from build123d import *

# Parameters (mm, degrees)
F0_R         = 19.3201303499
F1_DEPTH     = 45.72
F2_T1_DEPTH  = 55.325963316
F2_T3_DEPTH  = 52.1146440054
F2_T5_DEPTH  = 66.4513256331
F2_T7_DEPTH  = 30.5870827045
F2_T9_DEPTH  = 100.2395855595
F2_T11_DEPTH = 63.3652483976
F2_T13_DEPTH = 70.2836609721
F2_T15_DEPTH = 91.0933305156
F2_T20_DEPTH = 5.08
F2_T26_DEPTH = 5.08
F2_T36_DEPTH = 59.2845010847
F2_T41_DEPTH = 57.568004282
F2_T46_DEPTH = 31.0915483116
F2_T51_DEPTH = 75.0016446771
F2_T57_DEPTH = 59.2845010847
F2_T61_DEPTH = 57.568004282
F2_T68_DEPTH = 31.0915483116
F2_T72_DEPTH = 75.0016446771


# Not quite as in the source:
# - a fillet or chamfer that OpenCascade refuses, or shapes differently, is made with other operations: its cross-section is extruded or revolved along the edge and cut away or added


with BuildPart() as f1:
    # F0 (on Top) → F1 (new body)
    with BuildSketch(Plane.XY):
        Polygon((13.1280273199, 53.9313554764), (-58.0116845667, 30.691197142), (-58.1890903413, -7.2736367583), (-24.3045892566, -7.2736367583), (-13.1280263886, -56.7698441446), (25.1916181296, -42.0451648533), (19.1598236561, -19.8694467545), (68.3012157679, -26.610866189), (68.3012157679, 18.2727947831), align=None)
        with Locations((-4.6125496738, 20.4016622156)):
            Circle(F0_R, mode=Mode.SUBTRACT)
    extrude(amount=F1_DEPTH)

    # F2: fillet of radius 5.08 on 15 edges, made by hand

    # F2_s2 → F2_t1 (cut)
    with BuildSketch(Plane.XY.offset(-14.685963316)):
        with BuildLine():
            ThreePointArc((-14.4219236098, -51.039727833), (-11.8616097658, -54.4008391443), (-7.6445406789, -54.662763834))
            Line((-7.6445406789, -54.662763834), (-13.1280263886, -56.7698441446))
            Line((-13.1280263886, -56.7698441446), (-14.4219236098, -51.039727833))
        make_face()
    extrude(amount=F2_T1_DEPTH, mode=Mode.SUBTRACT)

    # F2_s4 → F2_t3 (cut)
    with BuildSketch(Plane.XY.offset(-11.4746440054)):
        with BuildLine():
            ThreePointArc((20.9071837297, -43.6914985622), (23.6160955732, -41.2464799373), (23.9869451943, -37.6162196147))
            Line((23.9869451943, -37.6162196147), (25.1916181296, -42.0451648533))
            Line((25.1916181296, -42.0451648533), (20.9071837297, -43.6914985622))
        make_face()
    extrude(amount=F2_T3_DEPTH, mode=Mode.SUBTRACT)

    # F2_s6 → F2_t5 (cut)
    with BuildSketch(Plane(origin=(-42.3016489373, -16.2548014713, 0), x_dir=(0, 0, 1), z_dir=(0.9334569329, 0.3586894958, 0))):
        with BuildLine():
            ThreePointArc((5.08, 48.2833194327), (1.4878975516, 46.7954218811), (0, 43.2033194327))
            Line((0, 43.2033194327), (0, 48.2833194327))
            Line((0, 48.2833194327), (5.08, 48.2833194327))
        make_face()
    extrude(amount=F2_T5_DEPTH, mode=Mode.SUBTRACT)

    # F2_s8 → F2_t7 (cut)
    with BuildSketch(Plane(origin=(-24.9632601794, -9.5923645646, 0), x_dir=(0, 0, 1), z_dir=(0.9334569329, 0.3586894958, 0))):
        with BuildLine():
            ThreePointArc((40.64, 48.2833194327), (44.2321024484, 46.7954218811), (45.72, 43.2033194327))
            Line((45.72, 43.2033194327), (45.72, 48.2833194327))
            Line((45.72, 48.2833194327), (40.64, 48.2833194327))
        make_face()
    extrude(amount=F2_T7_DEPTH, mode=Mode.SUBTRACT)

    # F2_s10 → F2_t9 (cut)
    with BuildSketch(Plane(origin=(39.8537401384, 13.0195527431, 0), x_dir=(0, 0, 1), z_dir=(-0.9505626114, -0.3105329641, 0))):
        with BuildLine():
            ThreePointArc((40.64, 47.1884448626), (44.2321024484, 45.700547311), (45.72, 42.1084448626))
            Line((45.72, 42.1084448626), (45.72, 47.1884448626))
            Line((45.72, 47.1884448626), (40.64, 47.1884448626))
        make_face()
    extrude(amount=F2_T9_DEPTH, mode=Mode.SUBTRACT)

    # F2_s12 → F2_t11 (cut)
    with BuildSketch(Plane(origin=(0.2014921201, 43.1193115962, 0), x_dir=(0, 0, 1), z_dir=(-0.0046728464, -0.9999890822, 0))):
        with BuildLine():
            ThreePointArc((40.64, 58.1544664567), (44.2321024484, 56.6665689051), (45.72, 53.0744664567))
            Line((45.72, 53.0744664567), (45.72, 58.1544664567))
            Line((45.72, 58.1544664567), (40.64, 58.1544664567))
        make_face()
    extrude(amount=F2_T11_DEPTH, mode=Mode.SUBTRACT)

    # F2_s14 → F2_t13 (cut)
    with BuildSketch(Plane.XZ.offset(-30.9727947831)):
        with BuildLine():
            ThreePointArc((68.3012157679, 40.64), (66.8133182163, 44.2321024484), (63.2212157679, 45.72))
            Line((63.2212157679, 45.72), (68.3012157679, 45.72))
            Line((68.3012157679, 45.72), (68.3012157679, 40.64))
        make_face()
    extrude(amount=F2_T13_DEPTH, mode=Mode.SUBTRACT)

    # F2_s16 → F2_t15 (cut)
    with BuildSketch(Plane(origin=(50.5132947185, -32.6468604807, 0), x_dir=(0, 0, 1), z_dir=(-0.8398598155, 0.5428033624, 0))):
        with BuildLine():
            ThreePointArc((40.64, 52.4207156327), (44.2321024484, 50.9328180811), (45.72, 47.3407156327))
            Line((45.72, 47.3407156327), (45.72, 52.4207156327))
            Line((45.72, 52.4207156327), (40.64, 52.4207156327))
        make_face()
    extrude(amount=F2_T15_DEPTH, mode=Mode.SUBTRACT)


with BuildPart() as f2_tool18:
    # F2_s19 → F2_t20 (new body)
    with BuildSketch(Plane.XY.offset(40.64)):
        Polygon((-9.4666833174, -49.9208026147), (-14.4219236098, -51.039727833), (-13.1280263886, -56.7698441446), (-7.6445406789, -54.662763834), align=None)
    extrude(amount=F2_T20_DEPTH)

    # F2_s21 → F2_t22 (revolve, cut)
    with BuildSketch(Plane(origin=(-9.4666833174, -49.9208026147, 40.64), x_dir=(0.4714422143, 0.8818969546, 0), z_dir=(0.8818969546, -0.4714422143, 0))):
        with BuildLine():
            ThreePointArc((0, -5.08), (5.08, 0), (0, 5.08))
            Line((0, 5.08), (0, -5.08))
        make_face()
    revolve(axis=Axis((-9.4666833174, -49.9208026147, 40.64), (0, 0, 1)), mode=Mode.SUBTRACT)


with BuildPart() as f1_1:
    add(f1.part)

    # F2_t17: cut F2_tool18
    add(f2_tool18.part, mode=Mode.SUBTRACT)


with BuildPart() as f2_tool24:
    # F2_s25 → F2_t26 (new body)
    with BuildSketch(Plane.XY.offset(40.64)):
        Polygon((19.0850410913, -38.9495373429), (20.9071837297, -43.6914985622), (25.1916181296, -42.0451648533), (23.9869451943, -37.6162196147), align=None)
    extrude(amount=F2_T26_DEPTH)

    # F2_s27 → F2_t28 (revolve, cut)
    with BuildSketch(Plane(origin=(19.0850410913, -38.9495373429, 40.64), x_dir=(-0.8919398586, 0.452154054, 0), z_dir=(0.452154054, 0.8919398586, 0))):
        with BuildLine():
            ThreePointArc((0, -5.08), (5.08, 0), (0, 5.08))
            Line((0, 5.08), (0, -5.08))
        make_face()
    revolve(axis=Axis((19.0850410913, -38.9495373429, 40.64), (0, 0, 1)), mode=Mode.SUBTRACT)


with BuildPart() as f1_2:
    add(f1_1.part)

    # F2_t23: cut F2_tool24
    add(f2_tool24.part, mode=Mode.SUBTRACT)

    # F2_s29 → F2_t30 (revolve, cut)
    with BuildSketch(Plane.XZ.offset(-20.4016622156)):
        with BuildLine():
            ThreePointArc((14.7075806761, 5.08), (16.1954782277, 1.4878975516), (19.7875806761, 0))
            Line((19.7875806761, 0), (14.7075806761, 0))
            Line((14.7075806761, 0), (14.7075806761, 5.08))
        make_face()
    revolve(axis=Axis((-4.6125496738, 20.4016622156, 0), (0, 0, 1)), mode=Mode.SUBTRACT)

    # F2_s31 → F2_t32 (revolve, cut)
    with BuildSketch(Plane.XZ.offset(-20.4016622156)):
        with BuildLine():
            ThreePointArc((14.7075806761, 40.64), (16.1954782277, 44.2321024484), (19.7875806761, 45.72))
            Line((19.7875806761, 45.72), (14.7075806761, 45.72))
            Line((14.7075806761, 45.72), (14.7075806761, 40.64))
        make_face()
    revolve(axis=Axis((-4.6125496738, 20.4016622156, 45.72), (0, 0, 1)), mode=Mode.SUBTRACT)


with BuildPart() as f2_tool34:
    # F2_s35 → F2_t36 (new body)
    with BuildSketch(Plane.YZ.offset(-70.8890903413)):
        with BuildLine():
            ThreePointArc((-7.2736367583, 40.64), (-5.7857392068, 44.2321024484), (-2.1936367583, 45.72))
            Line((-2.1936367583, 45.72), (-7.2736367583, 45.72))
            Line((-7.2736367583, 45.72), (-7.2736367583, 40.64))
        make_face()
    extrude(amount=F2_T36_DEPTH)

    split(bisect_by=Plane(origin=(-24.6882073851, -5.5747564614, 0), x_dir=(0, 0, 1), z_dir=(-0.9754410024, -0.2202608697, 0)), keep=Keep.TOP)


with BuildPart() as f1_3:
    add(f1_2.part)

    # F2_t33: cut F2_tool34
    add(f2_tool34.part, mode=Mode.SUBTRACT)


with BuildPart() as f2_tool39:
    # F2_s40 → F2_t41 (new body)
    with BuildSketch(Plane(origin=(-2.4136949173, 10.6892204341, 0), x_dir=(0, 0, 1), z_dir=(0.2202608697, -0.9754410024, 0))):
        with BuildLine():
            ThreePointArc((40.64, 25.3097904672), (44.2321024484, 23.8218929156), (45.72, 20.2297904672))
            Line((45.72, 20.2297904672), (45.72, 25.3097904672))
            Line((45.72, 25.3097904672), (40.64, 25.3097904672))
        make_face()
    extrude(amount=F2_T41_DEPTH)

    split(bisect_by=Plane.XZ.offset(7.2736367583), keep=Keep.TOP)


with BuildPart() as f1_4:
    add(f1_3.part)

    # F2_t38: cut F2_tool39
    add(f2_tool39.part, mode=Mode.SUBTRACT)


with BuildPart() as f2_tool44:
    # F2_s45 → F2_t46 (new body)
    with BuildSketch(Plane(origin=(11.1791797465, -41.0999313259, 0), x_dir=(0, 0, 1), z_dir=(-0.2624641197, 0.9649417526, 0))):
        with BuildLine():
            ThreePointArc((40.64, 13.2730969655), (44.2321024484, 11.7851994139), (45.72, 8.1930969655))
            Line((45.72, 8.1930969655), (45.72, 13.2730969655))
            Line((45.72, 13.2730969655), (40.64, 13.2730969655))
        make_face()
    extrude(amount=F2_T46_DEPTH)

    split(bisect_by=Plane(origin=(-2.3215052957, -16.9225491951, 0), x_dir=(0, 0, 1), z_dir=(-0.1359112078, -0.9907210221, 0)), keep=Keep.TOP)


with BuildPart() as f1_5:
    add(f1_4.part)

    # F2_t43: cut F2_tool44
    add(f2_tool44.part, mode=Mode.SUBTRACT)


with BuildPart() as f2_tool49:
    # F2_s50 → F2_t51 (new body)
    with BuildSketch(Plane(origin=(8.8991719713, -1.2208252209, 0), x_dir=(0, 0, 1), z_dir=(0.9907210221, -0.1359112078, 0))):
        with BuildLine():
            ThreePointArc((40.64, 17.0810438235), (44.2321024484, 15.5931462719), (45.72, 12.0010438235))
            Line((45.72, 12.0010438235), (45.72, 17.0810438235))
            Line((45.72, 17.0810438235), (40.64, 17.0810438235))
        make_face()
    extrude(amount=F2_T51_DEPTH)

    split(bisect_by=Plane(origin=(12.8077654479, 3.4837117113, 0), x_dir=(0, 0, 1), z_dir=(0.9649417526, 0.2624641197, 0)), keep=Keep.TOP)


with BuildPart() as f1_6:
    add(f1_5.part)

    # F2_t48: cut F2_tool49
    add(f2_tool49.part, mode=Mode.SUBTRACT)


with BuildPart() as f2_tool55:
    # F2_s56 → F2_t57 (new body)
    with BuildSketch(Plane.YZ.offset(-70.8890903413)):
        with BuildLine():
            ThreePointArc((-7.2736367583, 40.64), (-5.7857392068, 44.2321024484), (-2.1936367583, 45.72))
            Line((-2.1936367583, 45.72), (-7.2736367583, 45.72))
            Line((-7.2736367583, 45.72), (-7.2736367583, 40.64))
        make_face()
    extrude(amount=F2_T57_DEPTH)

    split(bisect_by=Plane(origin=(-24.6882073851, -5.5747564614, 0), x_dir=(0, 0, 1), z_dir=(0.9754410024, 0.2202608697, 0)), keep=Keep.TOP)


with BuildPart() as f2_tool59:
    # F2_s60 → F2_t61 (new body)
    with BuildSketch(Plane(origin=(-2.4136949173, 10.6892204341, 0), x_dir=(0, 0, 1), z_dir=(0.2202608697, -0.9754410024, 0))):
        with BuildLine():
            ThreePointArc((40.64, 25.3097904672), (44.2321024484, 23.8218929156), (45.72, 20.2297904672))
            Line((45.72, 20.2297904672), (45.72, 25.3097904672))
            Line((45.72, 25.3097904672), (40.64, 25.3097904672))
        make_face()
    extrude(amount=F2_T61_DEPTH)

    split(bisect_by=Plane.XZ.offset(7.2736367583), keep=Keep.BOTTOM)


with BuildPart() as f2_tool55_1:
    add(f2_tool55.part)

    # F2_t63: intersect F2_tool59
    add(f2_tool59.part, mode=Mode.INTERSECT)


with BuildPart() as f1_7:
    add(f1_6.part)

    # F2_t53: cut F2_tool55
    add(f2_tool55_1.part, mode=Mode.SUBTRACT)


with BuildPart() as f2_tool66:
    # F2_s67 → F2_t68 (new body)
    with BuildSketch(Plane(origin=(11.1791797465, -41.0999313259, 0), x_dir=(0, 0, 1), z_dir=(-0.2624641197, 0.9649417526, 0))):
        with BuildLine():
            ThreePointArc((40.64, 13.2730969655), (44.2321024484, 11.7851994139), (45.72, 8.1930969655))
            Line((45.72, 8.1930969655), (45.72, 13.2730969655))
            Line((45.72, 13.2730969655), (40.64, 13.2730969655))
        make_face()
    extrude(amount=F2_T68_DEPTH)

    split(bisect_by=Plane(origin=(-2.3215052957, -16.9225491951, 0), x_dir=(0, 0, 1), z_dir=(0.1359112078, 0.9907210221, 0)), keep=Keep.TOP)


with BuildPart() as f2_tool70:
    # F2_s71 → F2_t72 (new body)
    with BuildSketch(Plane(origin=(8.8991719713, -1.2208252209, 0), x_dir=(0, 0, 1), z_dir=(0.9907210221, -0.1359112078, 0))):
        with BuildLine():
            ThreePointArc((40.64, 17.0810438235), (44.2321024484, 15.5931462719), (45.72, 12.0010438235))
            Line((45.72, 12.0010438235), (45.72, 17.0810438235))
            Line((45.72, 17.0810438235), (40.64, 17.0810438235))
        make_face()
    extrude(amount=F2_T72_DEPTH)

    split(bisect_by=Plane(origin=(12.8077654479, 3.4837117113, 0), x_dir=(0, 0, 1), z_dir=(-0.9649417526, -0.2624641197, 0)), keep=Keep.TOP)


with BuildPart() as f2_tool66_1:
    add(f2_tool66.part)

    # F2_t74: intersect F2_tool70
    add(f2_tool70.part, mode=Mode.INTERSECT)


with BuildPart() as f1_8:
    add(f1_7.part)

    # F2_t64: cut F2_tool66
    add(f2_tool66_1.part, mode=Mode.SUBTRACT)


solid = f1_8.part
Design review of the part built by this model. Coordinates are the model's own, in mm. A direction names the side the tool comes from. Round coordinates to 2 decimals unless told otherwise and drop trailing zeros. Write each loop counter-clockwise with the first axis right and the second up, starting at its lowest first coordinate (ties: lowest second). Pieces come first, ordered by that corner, then holes.
Item 1: Draft analysis for pull direction X (two halves, no side actions). For faces 5 (the cylindrical face through (-11.92, -54.37, 20.04)), 6 (the cylindrical face through (-8.8, 1.54, 22.61)), 7 (the cylindrical face through (19.98, -28.39, 44.19)), 8 (the flat face through (-21.944, 42.474, 20.036)), state which applies: released by +X, released by -X, zero draft, split by the parting line, or undercut.
Item 2: For faces 1 (the flat face through (-41, -7.274, 20)), 2 (the cylindrical face through (-56.651, 11.968, 44.192)), 3 (the flat face through (21.61, -28.87, 20.04)), 4 (the cylindrical face through (-39.48, -5.83, 44.19)), list the 3-axis set-ups (+Z, -Z, +X, -X, +Y, -Y) from which the entire face can be reached by the end or side of a thin tool; tool diameter is ignored.
Item 3: Wall thickness on L1, parallel to X at y = 16.5, z = 35; L2, parallel to Y at x = 11, z = 33; L3, parallel to X at y = 13, z = 12: over which ranges is each line inside the solid? List them lowest first.
Item 4: Consider section A-A on z = 12. Give the boundary of the cut face in (x, y), and give its area (3 significant figures).
Item 5: For pin 1 Ø1 at (x, z) = (-12.5, 22.5) entering from +Y; pin 2 Ø2 at (x, z) = (-28.5, 18) entering from +Y; pin 3 Ø3 at (y, z) = (-11, 14) entering from -X, all flat-tipped, find the tip position at first contact; note any pin that passes through.
Check values:
1. face 5: split by the parting line
1. face 6: undercut
1. face 7: undercut
1. face 8: released by -X
2. face 1: +Z, -Z, -X, -Y
2. face 2: +Z, -X, +Y
2. face 3: +Z, -Z
2. face 4: +Z, -X, -Y
3. L1: x = -58.08 to -23.53, 14.31 to 68.3
3. L2: y = -47.5 to 9.02, 31.78 to 53.24
3. L3: x = -58.09 to -22.46, 13.23 to 68.3
4. outline: (-58.19, -7.27) - (-24.3, -7.27) - (-14.42, -51.04) arc R5.08 ccw to (-7.64, -54.66) - (20.91, -43.69) arc R5.08 ccw to (23.99, -37.62) - (19.16, -19.87) - (68.3, -26.61) - (68.3, 18.27) - (13.13, 53.93) - (-58.01, 30.69) - close; hole circle Ø38.64 at (-4.61, 20.4)
4. area: 7,270 mm2
5. pin 1: stops at y = 45.72
5. pin 2: stops at y = 40.66
5. pin 3: stops at x = -23.8
